from build123d import *

# Parameters (mm, degrees)
F0_W      = 27
F0_H      = 15.9
F0_W_2    = 15.9
F0_H_2    = 27
F0_W_3    = 3
F0_H_3    = 3
F1_DEPTH  = 21.9
F2_DEPTH  = 51.8
F3_R      = 7.95
F6_DEPTH  = 30
F7_DEPTH  = 30
F4_R      = 7.9
F8_DEPTH  = 30
F9_W      = 3.3
F9_H      = 3
F10_DEPTH = 51.9
F11_R     = 1.5


with BuildPart() as f1:
    # F0 (on Front) → F1 (new body)
    with BuildSketch(Plane.XZ):
        with BuildLine():
            Line((-34.3576915575, 15.9), (-42.3076915575, 15.9))
            Line((-42.3076915575, 15.9), (-42.3076915575, 7.9499999931))
            ThreePointArc((-42.3076915575, 7.9499999931), (-39.9791904704, 13.571498908), (-34.3576915575, 15.9))
        make_face()
        with BuildLine():
            ThreePointArc((-34.3576915575, 15.9), (-39.9791904704, 13.571498908), (-42.3076915575, 7.9499999931))
            ThreePointArc((-42.3076915575, 7.9499999931), (-39.9791904655, 2.3285010871), (-34.3576915575, 0))
            ThreePointArc((-34.3576915575, 0), (-28.7361926471, 2.3285010896), (-26.4076915575, 7.95))
            ThreePointArc((-26.4076915575, 7.95), (-28.7361926471, 13.5714989104), (-34.3576915575, 15.9))
        make_face()
        Polygon((-42.3076915575, 18.9), (-42.3076915575, 45.9), (-26.4076915575, 45.9), (-26.4076915575, 18.9), (-23.4076915575, 18.9), (-23.4076915575, 48.9), (-45.3076915575, 48.9), (-45.3076915575, 18.9), align=None)
        with Locations((-9.9076915575, 7.95)):
            Rectangle(F0_W, F0_H)
        with Locations((-34.3576915575, 32.4)):
            Rectangle(F0_W_2, F0_H_2)
        with BuildLine():
            ThreePointArc((-34.3576915575, 0), (-39.9791904655, 2.3285010871), (-42.3076915575, 7.9499999931))
            Line((-42.3076915575, 7.9499999931), (-42.3076915575, 0))
            Line((-42.3076915575, 0), (-34.3576915575, 0))
        make_face()
        with BuildLine():
            Line((-26.4076915575, 0), (-26.4076915575, 7.95))
            ThreePointArc((-26.4076915575, 7.95), (-28.7361926471, 2.3285010896), (-34.3576915575, 0))
            Line((-34.3576915575, 0), (-26.4076915575, 0))
        make_face()
        with BuildLine():
            Line((-26.4076915575, 7.95), (-26.4076915575, 15.9))
            Line((-26.4076915575, 15.9), (-34.3576915575, 15.9))
            ThreePointArc((-34.3576915575, 15.9), (-28.7361926471, 13.5714989104), (-26.4076915575, 7.95))
        make_face()
        Polygon((6.5923084425, 18.9), (-23.4076915575, 18.9), (-23.4076915575, 15.9), (3.5923084425, 15.9), (3.5923084425, 0), (-23.4076915575, 0), (-23.4076915575, -3), (6.5923084425, -3), align=None)
        Polygon((-26.4076915575, 18.9), (-42.3076915575, 18.9), (-42.3076915575, 15.9), (-34.3576915575, 15.9), (-26.4076915575, 15.9), align=None)
        Polygon((-23.4076915575, 15.9), (-26.4076915575, 15.9), (-26.4076915575, 7.95), (-26.4076915575, 0), (-23.4076915575, 0), align=None)
        Polygon((-42.3076915575, 15.9), (-42.3076915575, 18.9), (-45.3076915575, 18.9), (-45.3076915575, -3), (-23.4076915575, -3), (-23.4076915575, 0), (-26.4076915575, 0), (-34.3576915575, 0), (-42.3076915575, 0), (-42.3076915575, 7.9499999931), align=None)
        with Locations((-24.9076915575, 17.4)):
            Rectangle(F0_W_3, F0_H_3)
    extrude(amount=F1_DEPTH)

    # F0 (on Front) → F2 (join)
    with BuildSketch(Plane.XZ):
        Polygon((-42.3076915575, 15.9), (-42.3076915575, 18.9), (-45.3076915575, 18.9), (-45.3076915575, -3), (-23.4076915575, -3), (-23.4076915575, 0), (-26.4076915575, 0), (-34.3576915575, 0), (-42.3076915575, 0), (-42.3076915575, 7.9499999931), align=None)
        with BuildLine():
            ThreePointArc((-34.3576915575, 15.9), (-39.9791904704, 13.571498908), (-42.3076915575, 7.9499999931))
            ThreePointArc((-42.3076915575, 7.9499999931), (-39.9791904655, 2.3285010871), (-34.3576915575, 0))
            ThreePointArc((-34.3576915575, 0), (-28.7361926471, 2.3285010896), (-26.4076915575, 7.95))
            ThreePointArc((-26.4076915575, 7.95), (-28.7361926471, 13.5714989104), (-34.3576915575, 15.9))
        make_face()
        Polygon((-26.4076915575, 18.9), (-42.3076915575, 18.9), (-42.3076915575, 15.9), (-34.3576915575, 15.9), (-26.4076915575, 15.9), align=None)
        Polygon((-23.4076915575, 15.9), (-26.4076915575, 15.9), (-26.4076915575, 7.95), (-26.4076915575, 0), (-23.4076915575, 0), align=None)
        with Locations((-24.9076915575, 17.4)):
            Rectangle(F0_W_3, F0_H_3)
        with BuildLine():
            Line((-26.4076915575, 7.95), (-26.4076915575, 15.9))
            Line((-26.4076915575, 15.9), (-34.3576915575, 15.9))
            ThreePointArc((-34.3576915575, 15.9), (-28.7361926471, 13.5714989104), (-26.4076915575, 7.95))
        make_face()
        with BuildLine():
            Line((-34.3576915575, 15.9), (-42.3076915575, 15.9))
            Line((-42.3076915575, 15.9), (-42.3076915575, 7.9499999931))
            ThreePointArc((-42.3076915575, 7.9499999931), (-39.9791904704, 13.571498908), (-34.3576915575, 15.9))
        make_face()
        with BuildLine():
            ThreePointArc((-34.3576915575, 0), (-39.9791904655, 2.3285010871), (-42.3076915575, 7.9499999931))
            Line((-42.3076915575, 7.9499999931), (-42.3076915575, 0))
            Line((-42.3076915575, 0), (-34.3576915575, 0))
        make_face()
        with BuildLine():
            Line((-26.4076915575, 0), (-26.4076915575, 7.95))
            ThreePointArc((-26.4076915575, 7.95), (-28.7361926471, 2.3285010896), (-34.3576915575, 0))
            Line((-34.3576915575, 0), (-26.4076915575, 0))
        make_face()
    extrude(amount=F2_DEPTH)

    # F3 (on face) → F6 (cut)
    with BuildSketch(Plane.XZ.offset(51.8)):
        with Locations((-34.3576915575, 7.95)):
            Circle(F3_R)
    extrude(amount=-F6_DEPTH, mode=Mode.SUBTRACT)

    # F5 (on face) → F7 (cut)
    with BuildSketch(Plane.YZ.offset(6.5923084425)):
        with BuildLine():
            ThreePointArc((-3, 7.95), (-5.3285010896, 13.5714989104), (-10.95, 15.9))
            ThreePointArc((-10.95, 15.9), (-16.5714989104, 13.5714989104), (-18.9, 7.95))
            ThreePointArc((-18.9, 7.95), (-16.5714989104, 2.3285010896), (-10.95, 0))
            ThreePointArc((-10.95, 0), (-5.3285010896, 2.3285010896), (-3, 7.95))
        make_face()
    extrude(amount=-F7_DEPTH, mode=Mode.SUBTRACT)

    # F4 (on face) → F8 (cut)
    with BuildSketch(Plane.XY.offset(48.9)):
        with Locations((-34.3576915575, -10.9)):
            Circle(F4_R)
    extrude(amount=-F8_DEPTH, mode=Mode.SUBTRACT)

    # F9 (on face) → F10 (join)
    with BuildSketch(Plane(origin=(-45.3076915575, 0, 0), x_dir=(0, -1, 0), z_dir=(-1, 0, 0))):
        Polygon((3, -3), (0, -3), (0, -6.3), (0, -9.3), (16.3, -9.3), (16.3, -6.3), (3, -6.3), align=None)
        with Locations((-1.65, -7.8)):
            Rectangle(F9_W, F9_H)
        Polygon((-3.3, -9.3), (-3.3, -6.3), (-3.3, 7), (-6.3, 7), (-6.3, -9.3), align=None)
    extrude(amount=-F10_DEPTH)

    # F11
    f11_edges = [f1.edges().sort_by_distance(p)[0] for p in [
        (-45.307692, -9.65, -6.3),
        (6.592308, -9.65, -6.3),
        (-45.307692, 3.3, 0.35),
        (6.592308, 3.3, 0.35),
    ]]
    fillet(f11_edges, radius=F11_R)


solid = f1.part
Build history of the part. All positions in model axes, mm. A direction names the side the tool comes from. Give positions to 0.01 mm unless a question says otherwise; leave off trailing zeros. Order: outer loops, then holes, each group sorted by start corner. A loop starts at its lowest first (then second) coordinate and runs counter-clockwise, first axis right, second up. Notation, with made-up numbers: M 55,88 L 61,88 A17 ccw 61,101 Z; hole C -3.5,-37 d1. An arc over 180 degrees is marked long. Put each result on its own line as item: value.
Item 1: Drop flat-ended pins along their axis: pin 1 Ø4 at (x, z) = (1, 6.5) entering from -Y; pin 2 Ø1.4 at (x, z) = (-12, -5.5) entering from -Y; pin 3 Ø10.5 at (x, y) = (-17.5, -7) entering from +Z. Give the stop position or say it passes through.
Results are:
pin 1: y = -21.9
pin 2: y = -3
pin 3: z = 18.9
Item 2: Which spindle directions (+Z, -Z, +X, -X, +Y, -Y) get a long thin tool onto all of the face, cutting with end or side? Do faces 5 (the face through (-34, -21.8, 8)), 6 (the face through (-20, 5, 7)), 7 (the face through (-20, -10, -6.3)). Say none if no direction does.
Results are:
face 5: -Y
face 6: +Z, +X, -X, +Y
face 7: +X, -X, -Y
Item 3: Cut at A-A on x = -2. Write the cut outline in (y, z), then the cut area to 3 significant figures.
Results are:
outline: M -21.9,-3 L -3,-3 L -3,-6.3 L -16.3,-6.3 L -16.3,-9.3 L 6.3,-9.3 L 6.3,7 L 3.3,7 L 3.3,-6.3 L 0,-6.3 L 0,18.9 L -21.9,18.9 Z; hole C -10.95,7.95 d15.9
area: 399 mm2
Item 4: Cut at C-C on y = -39.5. Write the cut outline in (x, z).
Results are:
outline: M -45.31,-3 L -23.41,-3 L -23.41,18.9 L -45.31,18.9 Z; hole C -34.36,7.95 d15.9
Item 5: Pull direction Y, two halves, no side cores. Call faces 1 (the face through (-45.308, -16, 14)), 2 (the face through (-25, 0, 16)), 3 (the face through (-20, 2, -6.3)), 4 (the face through (-42, -51.8, 13)): +Y half, -Y half, draft (parallel to the pull), parting line (faces both ways), or undercut.
Results are:
face 1: draft
face 2: undercut
face 3: undercut
face 4: -Y half
Item 6: Cut at D-D on z = 35. Write the cut outline in (x, y), then the cut area to 3 significant figures.
Results are:
outline: M -45.31,-21.9 L -23.41,-21.9 L -23.41,0 L -45.31,0 Z; hole C -34.36,-10.9 d15.8
area: 284 mm2
Item 7: Wall check: probe 1 along Z at (x, y) = (-42, -8.5); probe 2 along Y at (x, z) = (-7.5, -6); probe 3 along Z at (x, y) = (-9.5, -13). Give the ranges that are in metal, low to high.
Results are:
probe 1: -9.3 to -6.3, -3 to 48.9
probe 2: -3 to 0, 3.3 to 6.3
probe 3: -9.3 to -6.3, -3 to 0.27, 15.63 to 18.9
Item 8: Cut at B-B on z = -5. Write the cut outline in (x, y).
Results are:
outline: M -45.31,-3 L 6.59,-3 L 6.59,0 L -45.31,0 Z; M -45.31,4.8 A1.5 ccw -43.81,3.3 L 5.09,3.3 A1.5 ccw 6.59,4.8 L 6.59,6.3 L -45.31,6.3 Z
